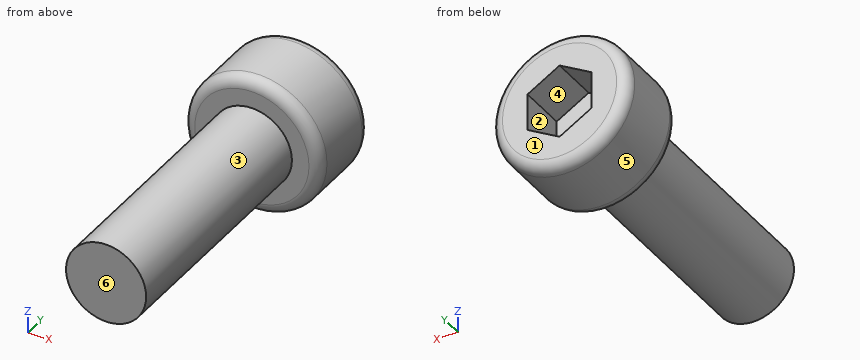
from build123d import *

# Parameters (mm, degrees)
F0_R     = 2.5
F1_DEPTH = 15
F0_R_2   = 4.265
F2_DEPTH = 5
F4_DEPTH = 3
F5_R     = 0.7


with BuildPart() as f1:
    # F0 (on Front) → F1 (new body)
    with BuildSketch(Plane.XZ):
        Circle(F0_R)
    extrude(amount=F1_DEPTH)

    # F0 (on Front) → F2 (join)
    with BuildSketch(Plane.XZ):
        Circle(F0_R_2)
        Circle(F0_R, mode=Mode.SUBTRACT)
        Circle(F0_R)
    extrude(amount=-F2_DEPTH)

    # F3 (on face) → F4 (cut)
    with BuildSketch(Plane(origin=(0, 5, 0), x_dir=(-1, 0, 0), z_dir=(0, 1, 0))):
        Polygon((2, 1.154701), (0, 2.309401), (-2, 1.154701), (-2, -1.154701), (0, -2.309401), (2, -1.154701), align=None)
    extrude(amount=-F4_DEPTH, mode=Mode.SUBTRACT)

    # F5
    f5_edges = [f1.edges().sort_by_distance(p)[0] for p in [
        (-4.265, 5, 0),
        (-4.265, 0, 0),
    ]]
    fillet(f5_edges, radius=F5_R)


solid = f1.part
The listing builds one solid part. Answer for the finished solid, in the listing's coordinates (mm). Face numbers are marked on the shaded views. A direction names the side the tool comes from. Coordinates: 2 decimals unless noted, no trailing zeros. Write each loop counter-clockwise with the first axis right and the second up, starting at its lowest first coordinate (ties: lowest second). Pieces come first, ordered by that corner, then holes. Notation, with made-up numbers: M 12,-10 L 62,-10 A10 cw 62,8 Z; hole C -7.75,15 d11. An arc over 180 degrees is marked long. Write each question's results on one line, items separated by ' | '.
Item 1: The part is cut by section B-B on y = -3.5. Determine the outline of the cut face in (x, z), and give its area (3 significant figures).
Answer below:
outline: C 0,0 d5 | area: 19.6 mm2
Item 2: Consider probe 1 along Z at (x, y) = (0, -12.5); probe 2 along Y at (x, z) = (-0.75, -3); probe 3 along Y at (x, z) = (-1, 0.25). Determine where each line is inside the solid, lowest interval first. Write a range as [from, to].
Answer below:
probe 1: [-2.5, 2.5] | probe 2: [0, 5] | probe 3: [-15, 2]
Item 3: Given P1, Ø1, axis at y = -12, z = 0.5, coming from the +X side; P2, Ø1, axis at y = -11, z = 1.5, coming from the -X side; P3, Ø1.5, axis at x = 2, y = -4.5, coming from the +Z side, each flat-ended and moving along its own axis, determine where each tip first touches the part or whether it passes through.
Answer below:
P1: x = 2.5 | P2: x = -2.29 | P3: z = 2.17
Item 4: For a pull along Z with two mould halves and no side action, classify the marked faces 4, 5 and 6 as released by +Z, released by -Z, zero draft, split by the parting line, or undercut.
Answer below:
face 4: undercut | face 5: split by the parting line | face 6: zero draft
Item 5: The part is cut by section A-A on z = 0. Determine the outline of the cut face in (x, y) (3 decimals), and give its area (3 significant figures).
Answer below:
outline: M -4.265,0.7 A0.7 ccw -3.565,0 L -2.5,0 L -2.5,-15 L 2.5,-15 L 2.5,0 L 3.565,0 A0.7 ccw 4.265,0.7 L 4.265,4.3 A0.7 ccw 3.565,5 L 2,5 L 2,2 L -2,2 L -2,5 L -3.565,5 A0.7 ccw -4.265,4.3 Z | area: 105 mm2
Item 6: Which of the six approach directions +Z, -Z, +X, -X, +Y, -Y give full straight-line access (tool end or side, diameter ignored) to the marked faces 1, 2 and 3?
Answer below:
face 1: +Z, -Z, +X, -X, +Y | face 2: +Y | face 3: -Y
